Design review of the part built by this model. Coordinates are the model's own, in mm. A direction names the side the tool comes from. Round coordinates to 2 decimals unless told otherwise and drop trailing zeros. Order: outer loops, then holes, each group sorted by start corner. A loop starts at its lowest first (then second) coordinate and runs counter-clockwise, first axis right, second up. Notation, with made-up numbers: M 21.25,-15 L 74.25,-15 A20 cw 74.25,18 Z; hole C 27,65 d2. An arc over 180 degrees is marked long. Write item = value, one per line. Start each with the question number.
Autodesk Inventor part; units mm, degrees
ref_plane "YZ Plane" through (0, 0, 0) normal (1, 0, 0) x (0, 1, 0)
ref_plane "XZ Plane" through (0, 0, 0) normal (0, 1, 0) x (-1, 0, 0)
ref_plane "XY Plane" through (0, 0, 0) normal (0, 0, 1) x (1, 0, 0)
sketch "Sketch1" plane through (0, 0, 0) normal (0, 0, 1) x (1, 0, 0)
  line L0 (0, 0) -> (25.4094, 0)
  line L1 (25.4094, 0) -> (25.4094, -355.6)
  line L2 (25.4094, -355.6) -> (0, -355.6)
  line L3 (0, -355.6) -> (0, 0)
  dimension "d0" = 355.6
extrude "Extrusion1" add sketch "Sketch1" along normal blind 6.35
fillet "Fillet1" radius 12.7 1 edges at (0, 0, 3.175)
fillet "Fillet2" radius 12.7 1 edges at (25.4094, 0, 3.175)
fillet "Fillet3" radius 12.7 1 edges at (25.4094, -355.6, 3.175)
fillet "Fillet4" radius 12.7 1 edges at (0, -355.6, 3.175)
shell "Shell1" thickness 2.54 removed faces 1 at (8.4698, -122.7667, 0)
shell "Shell2" thickness 2.54 removed faces 2 at (9.3165, -122.7667, 3.81) at (8.4698, -122.7667, 6.35)
properties part number "LiftWireLine14in"
(1) For faces 1 (the face through (19.972, -5.595, 3.219)), 2 (the face through (0, -180, 3)), list the 3-axis set-ups (+Z, -Z, +X, -X, +Y, -Y) from which the entire face can be reached by the end or side of a thin tool; tool diameter is ignored.
(2) Insertion check: pin 1 (12 mm diameter, centred on x = 9, y = -193, fed in from -Z) (1 decimal); pin 2 (1 mm diameter, centred on x = 22.5, z = 1.5, fed in from +Y). Each pin has a flat end and moves straight along its axis. Give the tip position at first contact, or say it passes through.
(3) Draft analysis for pull direction Y (two halves, no side actions). For faces 3 (the face through (3.62, -351.78, 3.22)), 4 (the face through (5.595, -5.437, 3.219)), 5 (the face through (25.409, -175, 3)), state which applies: pulls with the +Y half, pulls with the -Y half, needs draft (parallel to the pull), parting line crosses it, or undercut.
(4) Consider section B-B, the plane x = 6. Write out the cut boundary in (y, z).
(5) Consider section A-A, the plane y = -178.5. Write out the cut boundary in (x, z), then the cut area to 3 significant figures.
(6) For line 1 along X through (y, z) = (-319.5, 3.5); line 2 along Y through (x, z) = (13.5, 2.25); line 3 along Y through (x, z) = (11.5, 1.5), list the stretches that pass through material, from the lowest coordinate up. Write a range as [from, to].
Completed:
q1.face_1 = +Z, -Z
q1.face_2 = +Z, -Z, -X, +Y, -Y
q2.pin_1 = through
q2.pin_2 = -4.04
q3.face_3 = pulls with the -Y half
q3.face_4 = undercut
q3.face_5 = needs draft
q4.outline = M -353.69,0 L -350.54,0 L -350.54,6.35 L -353.69,6.35 Z; M -5.06,0 L -1.91,0 L -1.91,6.35 L -5.06,6.35 Z
q5.outline = M 0,0 L 2.54,0 L 2.54,6.35 L 0,6.35 Z; M 22.87,0 L 25.41,0 L 25.41,6.35 L 22.87,6.35 Z
q5.area = 32.3 mm2
q6.line_1 = [0, 2.54], [22.87, 25.41]
q6.line_2 = [-355.58, -353.03], [-2.57, -0.02]
q6.line_3 = [-355.54, -352.99], [-2.61, -0.06]
